Check sheet for the modelled part. Datum: model origin and axes. Units: mm. A direction names the side the tool comes from. Coordinates: 2 decimals unless noted, no trailing zeros. Write each loop counter-clockwise with the first axis right and the second up, starting at its lowest first coordinate (ties: lowest second). Pieces come first, ordered by that corner, then holes. Notation, with made-up numbers: M 63.25,46 L 117.25,46 A23 ccw 117.25,70 Z; hole C 73.5,30 d6. An arc over 180 degrees is marked long. Answer as CSV lines item,"result". Start each with the question number.
Q1. Sectioned sample at B-B, the plane y = -2.5. Count the separate pieces of the cut face and the enclosed holes in it, then the cut area to 3 significant figures.
Q2. Depth check by flat-ended pin: pin 1 Ø1 at (y, z) = (19, 3) entering from -X; pin 2 Ø6 at (x, y) = (-3.5, -6) entering from -Z; pin 3 Ø8 at (x, z) = (-26.5, 6) entering from -Y; pin 4 Ø5 at (x, y) = (-10.5, -1) entering from -Z. Enter the tip coordinate at first touch or a pass-through.
Q3. Thickness scan on line 1 along Z through (x, y) = (10.5, 19); line 2 along X through (y, z) = (22, -2); line 3 along Y through (x, z) = (-0.5, -2). Record the ranges inside material, lowest first. Write a range as from..to.
Q4. Sectioned sample at C-C, the plane y = 20. Record the cut outline in (x, z).
Q5. Access from +Z, -Z, +X, -X, +Y, -Y to the whole of each face (thin tool, end or side, straight path). Record for faces 1 (the cylindrical face through (4.586, 12.325, 0.264)), 2 (the flat face through (13, 25, 4)), 3 (the flat face through (-2.67, -10.88, -6.2)).
Q6. Sectioned sample at D-D, the plane z = -8. Record the cut outline in (x, y).
Q7. Mould release check, pull along Z, two halves, no side actions. Record for faces 4 (the cylindrical face through (6.084, 12.325, 0.198)), 5 (the flat face through (-33.69, -11.42, 4.47)), 6 (the cylindrical face through (-23.562, -10.903, -5.857)): pulls with the +Z half, pulls with the -Z half, needs draft (parallel to the pull), parting line crosses it, or undercut.
from build123d import *

# Parameters (mm, degrees)
F1_R        = 6
F1_R_2      = 4.5
F2_DEPTH    = 25
F2_FACE_R   = 6
F2_FACE_R_2 = 4.5
F4_R        = 9.5
F4_R_2      = 6
F4_R_3      = 4.5
F5_DEPTH    = 3
F6_R        = 6
F6_R_2      = 4.5
F7_DEPTH    = 4
F8_R        = 7
F8_R_2      = 6
F8_R_3      = 4.5
F9_DEPTH    = 7
F10_SIZE2   = 6
F10_SIZE    = 1
F11_R       = 6
F11_R_2     = 4.5
F12_DEPTH   = 20


with BuildPart() as f2:
    # F1 (on Front) → F2 (new body)
    with BuildSketch(Plane.XZ):
        with Locations((10.5797667056, 0)):
            Circle(F1_R)
        with Locations((10.5797667056, 0)):
            Circle(F1_R_2, mode=Mode.SUBTRACT)
    extrude(amount=-F2_DEPTH)

    # F3: sweep along a path in F0
    with BuildLine(Plane.XY) as f3_path:
        ThreePointArc((0, -4.9919255074), (3.3505289628, -3.4336417355), (4.7159582272, 0))
    # F2_face (on face) → F3 (sweep)
    with BuildSketch(Plane(origin=(10.5797667056, 0, 0), x_dir=(1, 0, 0), z_dir=(0, -1, 0))):
        Circle(F2_FACE_R)
        Circle(F2_FACE_R_2, mode=Mode.SUBTRACT)
    sweep(path=f3_path.line)

    # F4 (on face) → F5 (join)
    with BuildSketch(Plane(origin=(-0.2831251163, -0.0161098878, 0), x_dir=(0.0568083546, -0.9983851015, 0), z_dir=(-0.9983851015, -0.0568083546, 0))):
        with Locations((10.8476725327, 0)):
            Circle(F4_R)
        with Locations((10.8476725327, 0)):
            Circle(F4_R_2, mode=Mode.SUBTRACT)
        with Locations((10.8476725327, 0)):
            Circle(F4_R_2)
        with Locations((10.8476725327, 0)):
            Circle(F4_R_3, mode=Mode.SUBTRACT)
    extrude(amount=F5_DEPTH)

    # F6 (on face) → F7 (join)
    with BuildSketch(Plane(origin=(-3.2782804207, -0.1865349515, 0), x_dir=(0.0568083546, -0.9983851015, 0), z_dir=(-0.9983851015, -0.0568083546, 0))):
        with Locations((10.8476725327, 0)):
            Circle(F6_R)
        with Locations((10.8476725327, 0)):
            Circle(F6_R_2, mode=Mode.SUBTRACT)
    extrude(amount=F7_DEPTH)

    # F8 (on face) → F9 (join)
    with BuildSketch(Plane(origin=(-7.2718208266, -0.4137683698, 0), x_dir=(0.0568083546, -0.9983851015, 0), z_dir=(-0.9983851015, -0.0568083546, 0))):
        with Locations((10.8476725327, 0)):
            Circle(F8_R)
        with Locations((10.8476725327, 0)):
            Circle(F8_R_2, mode=Mode.SUBTRACT)
        with Locations((10.8476725327, 0)):
            Circle(F8_R_2)
        with Locations((10.8476725327, 0)):
            Circle(F8_R_3, mode=Mode.SUBTRACT)
    extrude(amount=F9_DEPTH)

    # F10
    f10_edges = [f2.edges().sort_by_distance(p)[0] for p in [
        (-14.041937, -4.652886, 0),
    ]]
    f10_side = f2.faces().sort_by_distance((-13.911163, -6.951178, 0))[0]
    chamfer(f10_edges, length=F10_SIZE, length2=F10_SIZE2, reference=f10_side)

    # F11 (on face) → F12 (join)
    with BuildSketch(Plane(origin=(-14.260516537, -0.8114268517, 0), x_dir=(0.0568083546, -0.9983851015, 0), z_dir=(-0.9983851015, -0.0568083546, 0))):
        with Locations((10.8476725327, 0)):
            Circle(F11_R)
        with Locations((10.8476725327, 0)):
            Circle(F11_R_2, mode=Mode.SUBTRACT)
    extrude(amount=F12_DEPTH)


solid = f2.part
Output:
1,separate pieces,"2"
1,enclosed holes,"1"
1,area,"77.8 mm^2"
2,pin 1,"stops at x = 5.13"
2,pin 2,"stops at z = -9.26"
2,pin 3,"stops at y = -18.06"
2,pin 4,"passes through"
3,line 1,"z = -6..-4.5, 4.5..6"
3,line 2,"x = 4.92..6.55, 14.61..16.24"
3,line 3,"y = -20.2..-14.93, -6.86..-1.59"
4,outline,"C 10.58,0 d12; hole C 10.58,0 d9"
5,face 1,"+Y"
5,face 2,"+Z, -Z, +X, -X, +Y"
5,face 3,"none"
6,outline,"M -2.95,-5.9 L -2.37,-16.13 L 0.62,-15.96 L 0.04,-5.73 Z"
7,face 4,"undercut"
7,face 5,"needs draft"
7,face 6,"parting line crosses it"
